Verification items for this drawing (mm, ordinates from the low corner). A direction names the side the tool comes from. Coordinates: 2 decimals unless noted, no trailing zeros. Order: outer loops, then holes, each group sorted by start corner. A loop starts at its lowest first (then second) coordinate and runs counter-clockwise, first axis right, second up. Notation, with made-up numbers: (-35, 79.5) - (16, 79.5) arc R30 ccw to (16, 115.5) - close; hole circle Ø1 at (85, 4.25). An arc over 180 degrees is marked (long way). Use CSV: the item, a comma, the result in double quotes. Start each with the question number.
1) Tool access check on the marked faces 4, 5 and 6. Record the directions out of +Z, -Z, +X, -X, +Y, -Y that give a thin tool (end or side, any length) a straight path to the whole face; none if there is none.
2) Draft check along Y on the marked faces 1, 2 and 3. Enter one of: released by +Y, released by -Y, zero draft, split by the parting line, or undercut.
3) Sectioned sample at A-A, the plane y = 49.5. Record the cut outline in (x, z) (1 decimal), and give its area (3 significant figures).
4) Thickness scan on probe 1 along X at (y, z) = (41.5, 19.5) (1 decimal); probe 2 along X at (y, z) = (70, 11) (1 decimal); probe 3 along Z at (x, y) = (10, 56) (1 decimal). Record the ranges inside material, lowest first. Write a range as [from, to].
5) Sectioned sample at C-C, the plane y = 9.5. Record the cut outline in (x, z) (1 decimal), and give its area (3 significant figures).
6) Depth check by flat-ended pin: P1, Ø12.5, axis at x = 18, y = 40.5, coming from the +Z side; P2, Ø1, axis at y = 71.5, z = 27.5, coming from the +X side; P3, Ø6.5, axis at y = 58, z = 24, coming from the -X side. Enter the tip coordinate at first touch or a pass-through.
7) Sectioned sample at B-B, the plane x = 79.5. Record the cut outline in (y, z).
8) Sectioned sample at D-D, the plane z = 20. Record the cut outline in (x, y).
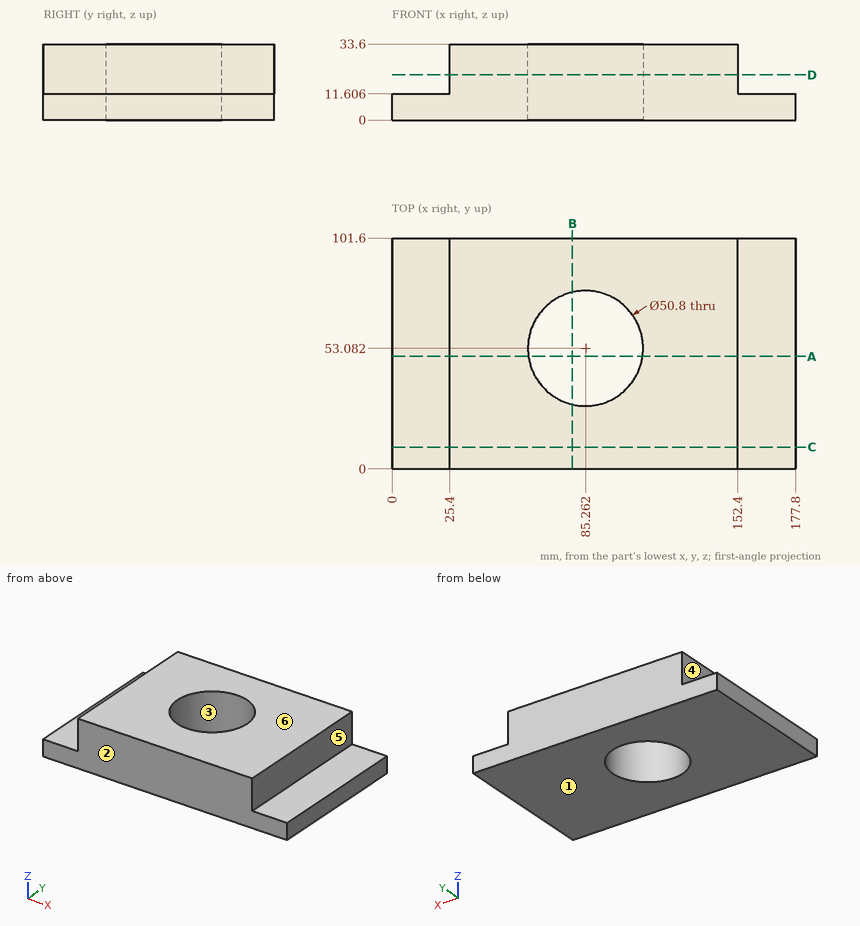
Evaluation:
1,face 4,"+Z, -X, +Y, -Y"
1,face 5,"+Z, +X, +Y, -Y"
1,face 6,"+Z, +X, -X, +Y, -Y"
2,face 1,"zero draft"
2,face 2,"released by -Y"
2,face 3,"undercut"
3,outline,"(0, 0) - (60.1, 0) - (60.1, 33.6) - (25.4, 33.6) - (25.4, 11.6) - (0, 11.6) - close; (110.4, 0) - (177.8, 0) - (177.8, 11.6) - (152.4, 11.6) - (152.4, 33.6) - (110.4, 33.6) - close"
3,area,"3,170 mm²"
4,probe 1,"[25.4, 62.7], [107.9, 152.4]"
4,probe 2,"[0, 66.3], [104.2, 177.8]"
4,probe 3,"[0, 11.6]"
5,outline,"(0, 0) - (177.8, 0) - (177.8, 11.6) - (152.4, 11.6) - (152.4, 33.6) - (25.4, 33.6) - (25.4, 11.6) - (0, 11.6) - close"
5,area,"4,860 mm²"
6,P1,"z = 11.61"
6,P2,"x = 152.4"
6,P3,"x = 25.4"
7,outline,"(0, 0) - (28.34, 0) - (28.34, 33.6) - (0, 33.6) - close; (77.82, 0) - (101.6, 0) - (101.6, 33.6) - (77.82, 33.6) - close"
8,outline,"(25.4, 0) - (152.4, 0) - (152.4, 101.6) - (25.4, 101.6) - close; hole circle Ø50.8 at (85.26, 53.08)"
